Input: dimensioned drawing with shaded views. Units: mm. Origin: part minimum x, y, z. A direction names the side the tool comes from. Give positions to 0.01 mm unless a question says otherwise; leave off trailing zeros. Write each loop counter-clockwise with the first axis right and the second up, starting at its lowest first coordinate (ties: lowest second). Pieces come first, ordered by that corner, then holes.
Q1. Reachability of the marked faces 1, 2 and 3 from +Z, -Z, +X, -X, +Y, -Y: full face, straight path, thin tool, end or side. Return the list, or none.
Q2. Pin query (flat end, axial travel): pin 1 Ø1 at (x, z) = (14.5, 2.5) entering from -Y; pin 2 Ø0.9 at (x, z) = (19, 2) entering from +Y. Return the tip coordinate at first contact, or that it passes through.
Q3. Section C-C (x = 19.75). Return the cut outline in (y, z).
Q4. Line query: line 1 (Y direction, x = 22.25, z = 1.9); line 2 (Y direction, x = 2.75, z = 0.6); line 3 (X direction, y = 14.25, z = 1.75) (3 decimals). Output: solid intervals per line, ascending.
Q5. Section B-B (x = 2.75). Return the cut outline in (y, z).
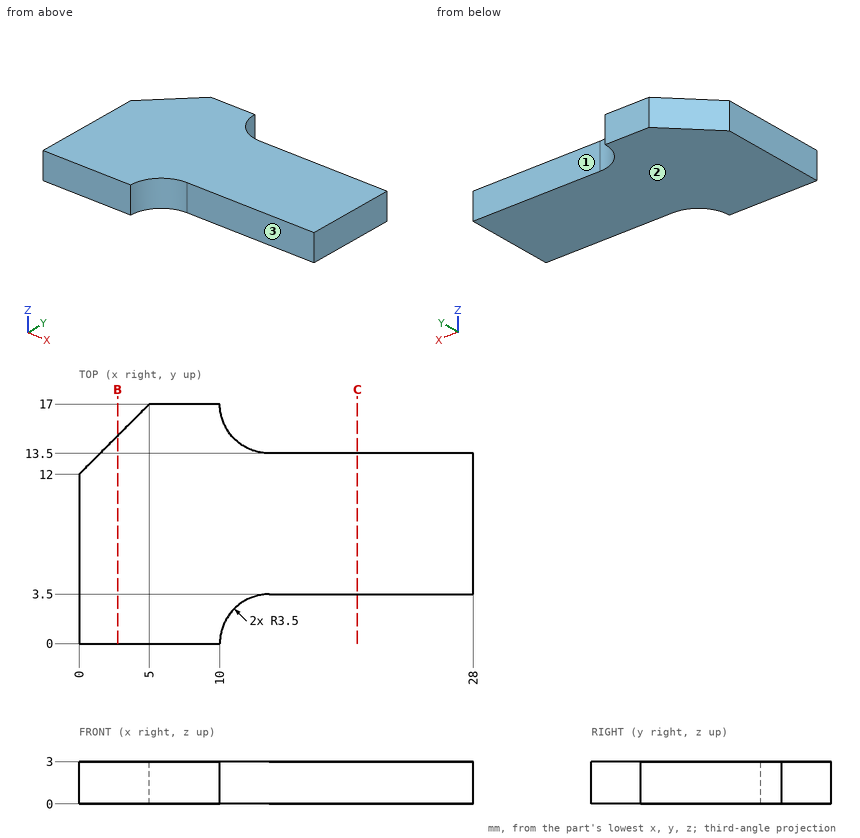
Computed:
1. face 1: +Z, -Z, +X, +Y
1. face 2: -Z, +X, -X, +Y, -Y
1. face 3: +Z, -Z, +X, -Y
2. pin 1: stops at y = 3.5
2. pin 2: stops at y = 13.5
3. outline: (3.5, 0) - (13.5, 0) - (13.5, 3) - (3.5, 3) - close
4. line 1: y = 3.5 to 13.5
4. line 2: y = 0 to 14.75
4. line 3: x = 2.25 to 11.335
5. outline: (0, 0) - (14.75, 0) - (14.75, 3) - (0, 3) - close
